```python
from build123d import *

# Parameters (mm, degrees)
SKETCH1_R           = 50
SKETCH1_R_2         = 1.475
SKETCH1_R_3         = 2.6
BOSS_EXTRUDE1_DEPTH = 4
SKETCH2_R           = 1.5
CUT_EXTRUDE1_DEPTH  = 10
BOSS_EXTRUDE3_DEPTH = 9.1
CIRPATTERN1_COUNT   = 4
CUT_EXTRUDE2_START  = -3
CUT_EXTRUDE2_DEPTH  = 5
CUT_EXTRUDE3_DEPTH  = 15
CIRPATTERN2_COUNT   = 4
CIRPATTERN3_COUNT   = 4
BOSS_EXTRUDE4_START = -4
SKETCH11_R          = 2.6
SKETCH11_R_2        = 1.475
SKETCH11_R_3        = 2.656466029
BOSS_EXTRUDE4_DEPTH = 4
SKETCH12_R          = 2.5
CUT_EXTRUDE4_DEPTH  = 10
CIRPATTERN4_COUNT   = 4


with BuildPart() as part:
    # Sketch1 → Boss-Extrude1 (new body)
    with BuildSketch(Plane(origin=(0, 0, 0), x_dir=(1, 0, 0), z_dir=(0, 1, 0))):
        with Locations(Location((0, 0, 0), (0, 0, 270))):
            Circle(SKETCH1_R)
        with Locations(Location((0, 13, 0), (0, 0, 270))):
            Circle(SKETCH1_R_2, mode=Mode.SUBTRACT)
        with Locations(Location((11.258330249, 6.5, 0), (0, 0, 270))):
            Circle(SKETCH1_R_2, mode=Mode.SUBTRACT)
        with Locations(Location((11.258330249, -6.5, 0), (0, 0, 270))):
            Circle(SKETCH1_R_2, mode=Mode.SUBTRACT)
        with Locations(Location((0, -13, 0), (0, 0, 270))):
            Circle(SKETCH1_R_2, mode=Mode.SUBTRACT)
        with Locations(Location((-11.258330249, -6.5, 0), (0, 0, 270))):
            Circle(SKETCH1_R_2, mode=Mode.SUBTRACT)
        with Locations(Location((-11.258330249, 6.5, 0), (0, 0, 270))):
            Circle(SKETCH1_R_2, mode=Mode.SUBTRACT)
        with Locations(Location((-24.148145657, 6.470476128, 0), (0, 0, 270))):
            Circle(SKETCH1_R_3, mode=Mode.SUBTRACT)
        with Locations(Location((6.470476128, 24.148145657, 0), (0, 0, 270))):
            Circle(SKETCH1_R_3, mode=Mode.SUBTRACT)
        with Locations(Location((24.148145657, -6.470476128, 0), (0, 0, 270))):
            Circle(SKETCH1_R_3, mode=Mode.SUBTRACT)
        with Locations(Location((-6.470476128, -24.148145657, 0), (0, 0, 270))):
            Circle(SKETCH1_R_3, mode=Mode.SUBTRACT)
    extrude(amount=BOSS_EXTRUDE1_DEPTH)

    # Sketch2 → Cut-Extrude1 (cut)
    with BuildSketch(Plane(origin=(0, 4, 0), x_dir=(1, 0, 0), z_dir=(0, 1, 0))):
        with Locations((-25, 43.301270189)):
            Circle(SKETCH2_R)
    extrude(amount=-CUT_EXTRUDE1_DEPTH, mode=Mode.SUBTRACT)

    # Sketch8 → Boss-Extrude3 (add)
    with BuildSketch(Plane(origin=(0, 4, 0), x_dir=(1, 0, 0), z_dir=(0, 1, 0))):
        Polygon((-6.906956469, 23.263199529), (-11.8, 20.438199529), (-8.2, 14.202816622), (-3.306956469, 17.027816622), align=None)
        Polygon((-8.2, 14.202816622), (-11.8, 20.438199529), (-16.693043531, 17.613199529), (-13.093043531, 11.377816622), align=None)
    boss_extrude3 = extrude(amount=BOSS_EXTRUDE3_DEPTH)

    # CirPattern1: Boss-Extrude3 ×4 about axis
    cirpattern1_axis = Axis((0, 0, 0), (0, 1, 0))
    for i in range(1, CIRPATTERN1_COUNT):
        add(boss_extrude3.rotate(cirpattern1_axis, i * 360 / CIRPATTERN1_COUNT))

    # Sketch9 → Cut-Extrude2 (cut)
    with BuildSketch(Plane(origin=(-11.8, 0, -20.438199529), x_dir=(-0.8660254037844384, 0, 0.5000000000000006), z_dir=(-0.5000000000000006, 0, -0.8660254037844384)).offset(CUT_EXTRUDE2_START)):
        Polygon((0, 5.3), (0, 12.7), (-2.136195996, 12.7), (-4.272391992, 9), (-2.136195996, 5.3), align=None)
        Polygon((2.136195996, 12.7), (0, 12.7), (0, 5.3), (2.136195996, 5.3), (4.272391992, 9), align=None)
        Polygon((0, 12.7), (0, 13.1), (-4.272391992, 13.1), (-4.272391992, 9), (-2.136195996, 12.7), align=None)
        Polygon((4.272391992, 13.1), (0, 13.1), (0, 12.7), (2.136195996, 12.7), (4.272391992, 9), align=None)
    cut_extrude2 = extrude(amount=-CUT_EXTRUDE2_DEPTH, mode=Mode.SUBTRACT)

    # Sketch10 → Cut-Extrude3 (cut)
    with BuildSketch(Plane(origin=(-11.8, 0, -20.438199529), x_dir=(-0.8660254037844384, 0, 0.5000000000000006), z_dir=(-0.5000000000000006, 0, -0.8660254037844384))):
        with BuildLine():
            ThreePointArc((2.1, 9), (1.48492424, 10.48492424), (0, 11.1))
            Line((0, 11.1), (0, 6.9))
            ThreePointArc((0, 6.9), (1.48492424, 7.51507576), (2.1, 9))
        make_face()
        with BuildLine():
            Line((0, 6.9), (0, 11.1))
            ThreePointArc((0, 11.1), (-2.1, 9), (0, 6.9))
        make_face()
    cut_extrude3 = extrude(amount=-CUT_EXTRUDE3_DEPTH, mode=Mode.SUBTRACT)

    # CirPattern2: Cut-Extrude2 ×4 about axis
    cirpattern2_axis = Axis((0, 0, 0), (0, 1, 0))
    for i in range(1, CIRPATTERN2_COUNT):
        add(cut_extrude2.rotate(cirpattern2_axis, i * 360 / CIRPATTERN2_COUNT), mode=Mode.SUBTRACT)

    # CirPattern3: Cut-Extrude3 ×4 about axis
    cirpattern3_axis = Axis((0, 4, 0), (0, 1, 0))
    for i in range(1, CIRPATTERN3_COUNT):
        add(cut_extrude3.rotate(cirpattern3_axis, i * 360 / CIRPATTERN3_COUNT), mode=Mode.SUBTRACT)

    # Sketch11 → Boss-Extrude4 (add)
    with BuildSketch(Plane(origin=(0, 4, 0), x_dir=(1, 0, 0), z_dir=(0, 1, 0)).offset(BOSS_EXTRUDE4_START)):
        with Locations((-24.148145657, 6.470476128)):
            Circle(SKETCH11_R)
        with Locations((-6.470476128, -24.148145657)):
            Circle(SKETCH11_R)
        with Locations((0, -13)):
            Circle(SKETCH11_R_2)
        with Locations((-11.258330249, -6.5)):
            Circle(SKETCH11_R_2)
        with Locations((24.148145657, -6.470476128)):
            Circle(SKETCH11_R_3)
        with Locations((6.470476128, 24.148145657)):
            Circle(SKETCH11_R)
        with Locations((0, 13)):
            Circle(SKETCH11_R_2)
        with Locations((11.258330249, 6.5)):
            Circle(SKETCH11_R_2)
        with Locations((11.258330249, -6.5)):
            Circle(SKETCH11_R_2)
        with Locations((-11.258330249, 6.5)):
            Circle(SKETCH11_R_2)
        with BuildLine():
            ThreePointArc((-26.287641956, 42.531868997), (-25.021511025, 43.338528377), (-23.689858044, 44.031700238))
            ThreePointArc((-23.689858044, 44.031700238), (-24.25, 42.002232084), (-26.287641956, 42.531868997))
        make_face()
    extrude(amount=BOSS_EXTRUDE4_DEPTH)

    # Sketch12 → Cut-Extrude4 (cut)
    with BuildSketch(Plane(origin=(0, 4, 0), x_dir=(1, 0, 0), z_dir=(0, 1, 0))):
        with Locations(Location((36.861841993, -25.810939636, 0), (0, 0, 270))):
            Circle(SKETCH12_R)
    cut_extrude4 = extrude(amount=-CUT_EXTRUDE4_DEPTH, mode=Mode.SUBTRACT)

    # CirPattern4: Cut-Extrude4 ×4 about axis
    cirpattern4_axis = Axis((0, 0, 0), (0, 1, 0))
    for i in range(1, CIRPATTERN4_COUNT):
        add(cut_extrude4.rotate(cirpattern4_axis, i * 360 / CIRPATTERN4_COUNT), mode=Mode.SUBTRACT)


solid = part.part
```
Input: part model. Units: mm. Frame: model coordinates. A direction names the side the tool comes from. Give positions to 0.01 mm unless a question says otherwise; leave off trailing zeros. Order: outer loops, then holes, each group sorted by start corner. A loop starts at its lowest first (then second) coordinate and runs counter-clockwise, first axis right, second up. Notation, with made-up numbers: M 15.5,40 L 44.5,40 A33 cw 44.5,70 Z; hole C -17.5,73 d10. An arc over 180 degrees is marked long. Return JSON: item names as keys, results as strings.
1) Section query B-B on z = 0. Output: boundary loops of the cut face in (x, y), and give its area (3 significant figures).
Taken from the geometry:
{"outline": "M -50,0 L 50,0 L 50,4 L -50,4 Z", "area": "400 mm2"}
2) Contact query for flat-ended pins moving along their axis: pin 1 (3 mm diameter, centred on x = 3.5, y = 9, fed in from -Z); pin 2 (1.5 mm diameter, centred on y = 7, z = 13.5, fed in from +X); pin 3 (6.5 mm diameter, centred on x = -25.81, z = 36.86, fed in from +Y). Output: stop coordinate, or through.
Taken from the geometry:
{"pin 1": "stops at z = 16.14", "pin 2": "stops at x = 14.75", "pin 3": "stops at y = 4"}
3) Section query C-C on z = 33. Output: boundary loops of the cut face in (x, y), and give its area (3 significant figures).
Taken from the geometry:
{"outline": "M -37.56,0 L 37.56,0 L 37.56,4 L -37.56,4 Z", "area": "301 mm2"}
4) Access query for faces 5 (the face through (-11.73, 6.46, -20.48)), 6 (the face through (14.163, 4.442, -8.269)), 7 (the face through (-5.08, 8.49, -20.1)). Directions: +Z, -Z, +X, -X, +Y, -Y. A direction counts if a zero-diameter tool reaches every point of the face in a straight line with its end or side. Return the directions, or none.
Taken from the geometry:
{"face 5": "-Z, -X, +Y", "face 6": "+Y", "face 7": "-Z, +X, +Y"}
5) Line query: L1, parallel to Y at x = 39, z = -13; L2, parallel to Z at x = -15, y = 8; L3, parallel to Z at x = 26.5, y = 2.25 (3 decimals). Output: solid intervals per line, ascending. Write a range as [from, to].
Taken from the geometry:
{"L1": "y = [0, 4]", "L2": "z = [-18.59, -14.68], [12.93, 15.18]", "L3": "z = [-42.4, -39.265], [-34.459, 42.4]"}
6) Mould query, pull axis Z, two halves, no side actions, for faces 1 (the face through (-5.565, 11.079, -18.183)), 2 (the face through (6.477, 7.176, 17.657)), 3 (the face through (12.027, 7.124, 14.452)), 4 (the face through (18.82, 10.12, -8.6)). Classes: released by +Z, released by -Z, zero draft, split by the parting line, or undercut.
Taken from the geometry:
{"face 1": "released by +Z", "face 2": "released by -Z", "face 3": "undercut", "face 4": "undercut"}
7) Section query A-A on z = -26.5. Output: boundary loops of the cut face in (x, y) (3 decimals), and give its area (3 significant figures).
Taken from the geometry:
{"outline": "M -42.4,0 L -39.265,0 L -39.265,4 L -42.4,4 Z; M -34.459,0 L 42.4,0 L 42.4,4 L -34.459,4 Z", "area": "320 mm2"}
